Study the drawing (mm; zero at the part's minimum x, y, z) and answer. A direction names the side the tool comes from. Give positions to 0.01 mm unless a question says otherwise; leave off trailing zeros. Loops run counter-clockwise (first coordinate to the right, second up) from the corner with the lowest first, then second, coordinate; pieces in that order, holes last. Notation, with made-up numbers: (-28.5, -32.75) - (-2.5, -32.75) arc R23 cw to (-2.5, -21.75) - close; hole circle Ø9 at (-5.75, 50). An arc over 180 degrees is marked (long way). One line per item, written item: value. Start each with the question number.
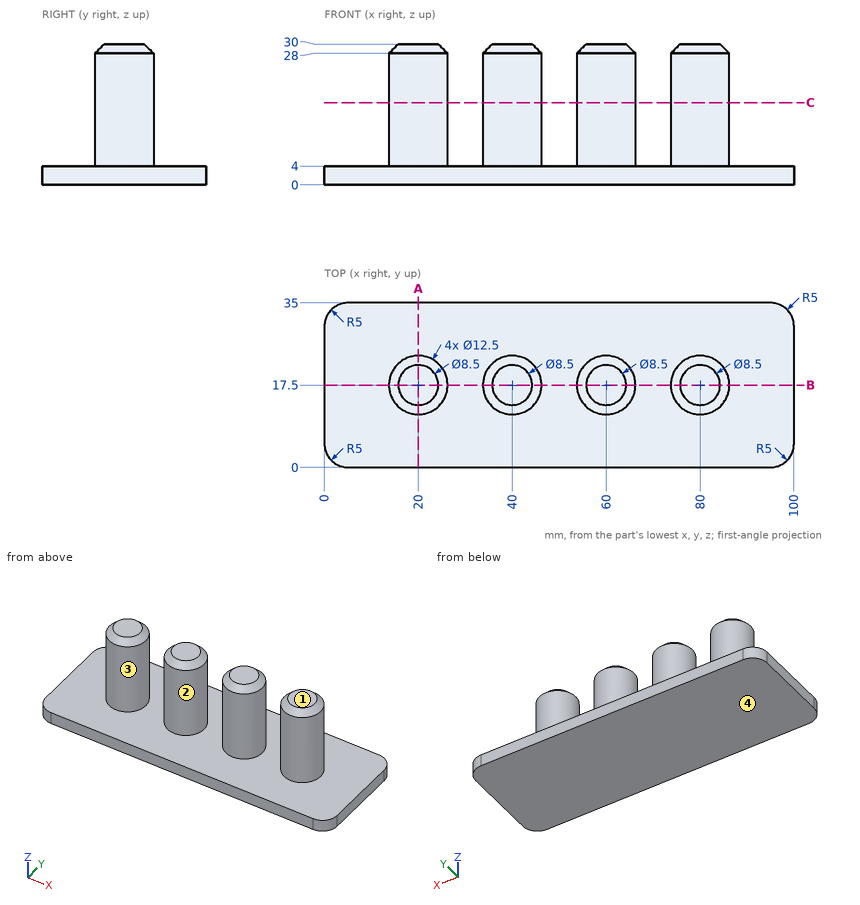
1. Flat-ended cylindrical pins translate along their axes: pin 1 (6 mm diameter, centred on y = 11, z = 16, fed in from +X); pin 2 (10 mm diameter, centred on y = 27.5, z = 12.5, fed in from +X); pin 3 (4 mm diameter, centred on x = 19, y = 9.5, fed in from -Z); pin 4 (4 mm diameter, centred on y = 26, z = 15, fed in from +X). Find the tip coordinate at first contact, or state that the pin passes through.
2. For the marked faces 1 and 2, determine the directions among +Z, -Z, +X, -X, +Y, -Y from which every point of the face is accessible in a straight line to the end or side of a thin tool.
3. Determine the mould class of the marked faces 3 and 4 for opening direction X: released by +X, released by -X, zero draft, split by the parting line, or undercut.
4. A cutting plane is placed at B-B (y = 17.5). Determine the outline of the cut face in (x, z), plus the area to 3 significant figures.
5. Find the intervals of material crossed by L1, parallel to X at y = 19, z = 23.5; L2, parallel to X at y = 23, z = 6.5; L3, parallel to Z at x = 11.5, y = 9.5, in increasing order. Write a range as [from, to].
6. A cutting plane is placed at A-A (x = 20). Determine the outline of the cut face in (y, z).
7. A cutting plane is placed at C-C (z = 17.5). Determine the outline of the cut face in (x, y).
Results below:
1. pin 1: stops at x = 85.18
1. pin 2: stops at x = 83.75
1. pin 3: stops at z = 0
1. pin 4: passes through
2. face 1: +Z, +X, -X, +Y, -Y
2. face 2: +Z
3. face 3: undercut
3. face 4: zero draft
4. outline: (0, 0) - (100, 0) - (100, 4) - (86.25, 4) - (86.25, 28) - (84.25, 30) - (75.75, 30) - (73.75, 28) - (73.75, 4) - (66.25, 4) - (66.25, 28) - (64.25, 30) - (55.75, 30) - (53.75, 28) - (53.75, 4) - (46.25, 4) - (46.25, 28) - (44.25, 30) - (35.75, 30) - (33.75, 28) - (33.75, 4) - (26.25, 4) - (26.25, 28) - (24.25, 30) - (15.75, 30) - (13.75, 28) - (13.75, 4) - (0, 4) - close
4. area: 1,680 mm^2
5. L1: x = [13.93, 26.07], [33.93, 46.07], [53.93, 66.07], [73.93, 86.07]
5. L2: x = [17.03, 22.97], [37.03, 42.97], [57.03, 62.97], [77.03, 82.97]
5. L3: z = [0, 4]
6. outline: (0, 0) - (35, 0) - (35, 4) - (23.75, 4) - (23.75, 28) - (21.75, 30) - (13.25, 30) - (11.25, 28) - (11.25, 4) - (0, 4) - close
7. outline: circle Ø12.5 at (20, 17.5); circle Ø12.5 at (40, 17.5); circle Ø12.5 at (60, 17.5); circle Ø12.5 at (80, 17.5)
